Here's how the part is built. I have some questions about the finished solid (model axes, mm). Face numbers are marked on the shaded views. Give positions to 0.01 mm unless a question says otherwise; leave off trailing zeros. Loops run counter-clockwise (first coordinate to the right, second up) from the corner with the lowest first, then second, coordinate; pieces in that order, holes last. Notation, with made-up numbers: M -37,73 L 19,73 A19 ccw 19,95 Z; hole C -19.5,-34.75 d7. An arc over 180 degrees is marked long. Answer as CSV lines item,"result". Start each with the question number.
Item 1: I want a section at C-C on z = -1.75. List the corners of the cut face in (x, y) for me.
Item 2: I want a section at A-A on y = 0. List the corners of the cut face in (x, z) for me, plus the area to 3 significant figures.
Item 3: If we mould it in two halves opening along Z, with no side actions, what happens to the marked faces 1, 2 and 3? For each: released by +Z, released by -Z, zero draft, split by the parting line, or undercut.
Item 4: If I drill on line 1 along Z through (x, y) = (-1.85, 0.9); line 2 along X through (y, z) = (0.05, -1.75); line 3 along Y through (x, z) = (-0.2, 1), over which ranges is the centre line in solid material (lowest first)? Write a range as from..to.
Item 5: I want a section at B-B on x = 0. List the corners of the cut face in (y, z) for me.
Item 6: Will these pins go through, and if not, where does the flat tip stop? P1, Ø0.6, axis at x = -0.5, z = 1.5, coming from the -Y side; P2, Ø1.5, axis at x = 1, z = -2.5, coming from the +Y side; P3, Ø0.6, axis at x = 1, y = 0, coming from the +Z side.
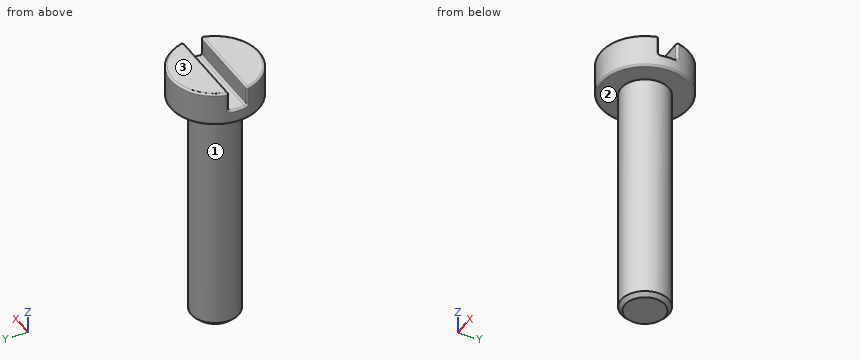
from build123d import *

# Parameters (mm, degrees)
SKIZZE2_W                       = 4.5
SKIZZE2_H                       = 0.9
SCHNITT_LINEAR_AUSTRAGEN1_DEPTH = 1
FASE1_SIZE                      = 0.2
VERRUNDUNG2_R                   = 0.1


with BuildPart() as part:
    # Skizze1 → Rotation1 (revolve)
    with BuildSketch(Plane(origin=(0, 0, 0), x_dir=(0, 0, -1), z_dir=(1, 0, 0))):
        Polygon((-1.7, 0), (-1.7, 2.25), (0, 2.25), (0, 1.21), (12, 1.21), (12, 0), align=None)
    revolve(axis=Axis((0, 0, 21.919879518), (0, 0, -1)))

    # Skizze2 → Schnitt-Linear austragen1 (cut)
    with BuildSketch(Plane.XY.offset(1.7)):
        Rectangle(SKIZZE2_W, SKIZZE2_H)
    extrude(amount=-SCHNITT_LINEAR_AUSTRAGEN1_DEPTH, mode=Mode.SUBTRACT)

    # Fase1
    fase1_edges = [part.edges().sort_by_distance(p)[0] for p in [
        (0, -1.21, -12),
    ]]
    chamfer(fase1_edges, length=FASE1_SIZE)

    # Verrundung2
    verrundung2_edges = [part.edges().sort_by_distance(p)[0] for p in [
        (1.423024947, 1.742842506, 1.7),
        (0, -2.25, 1.7),
        (2.25, 0, 0.7),
        (2.204540769, 0.45, 1.2),
        (2.204540769, -0.45, 1.2),
        (-2.25, 0, 0.7),
        (-2.204540769, 0.45, 1.2),
        (-2.204540769, -0.45, 1.2),
        (0, -0.45, 0.7),
        (0, 0.45, 0.7),
        (0, 0.45, 1.7),
        (0, -0.45, 1.7),
        (0, -2.25, 0),
    ]]
    fillet(verrundung2_edges, radius=VERRUNDUNG2_R)


solid = part.part
Result:
1,outline,"C 0,0 d2.42"
2,outline,"M -2.25,0.1 A0.1 ccw -2.15,0 L -1.21,0 L -1.21,-11.8 L -1.01,-12 L 1.01,-12 L 1.21,-11.8 L 1.21,0 L 2.15,0 A0.1 ccw 2.25,0.1 L 2.25,0.6 A0.1 ccw 2.15,0.7 L -2.15,0.7 A0.1 ccw -2.25,0.6 Z"
2,area,"32.1 mm^2"
3,face 1,"zero draft"
3,face 2,"released by -Z"
3,face 3,"released by +Z"
4,line 1,"0..1.7"
4,line 2,"-1.21..1.21"
4,line 3,"-2.24..-0.45, 0.45..2.24"
5,outline,"M -2.25,0.1 A0.1 ccw -2.15,0 L -1.21,0 L -1.21,-11.8 L -1.01,-12 L 1.01,-12 L 1.21,-11.8 L 1.21,0 L 2.15,0 A0.1 ccw 2.25,0.1 L 2.25,1.6 A0.1 ccw 2.15,1.7 L 0.55,1.7 A0.1 ccw 0.45,1.6 L 0.45,0.8 A0.1 cw 0.35,0.7 L -0.35,0.7 A0.1 cw -0.45,0.8 L -0.45,1.6 A0.1 ccw -0.55,1.7 L -2.15,1.7 A0.1 ccw -2.25,1.6 Z"
6,P1,"y = -2.24"
6,P2,"y = 1.18"
6,P3,"z = 0.7"
